CAD build for the part. Positions are in the model's coordinates, mm. Give positions to 0.01 mm unless a question says otherwise; leave off trailing zeros. Write each loop counter-clockwise with the first axis right and the second up, starting at its lowest first coordinate (ties: lowest second). Pieces come first, ordered by that corner, then holes. Notation, with made-up numbers: (54.5, 21.5) -> (71.5, 21.5) arc R31 ccw to (71.5, 49.5) -> close; hole circle Ø3 at (82.25, -31). An arc over 180 degrees is marked (long way). Answer as a JSON object with one key per item and string values.
Autodesk Inventor part; units mm, degrees
ref_plane "YZ Plane" through (0, 0, 0) normal (1, 0, 0) x (0, 1, 0)
ref_plane "XZ Plane" through (0, 0, 0) normal (0, 1, 0) x (-1, 0, 0)
ref_plane "XY Plane" through (0, 0, 0) normal (0, 0, 1) x (1, 0, 0)
sketch "Sketch1" plane through (0, 0, 0) normal (0, 1, 0) x (-1, 0, 0)
  line L0 (0, 0) -> (254, 0)
  line L1 (0, -25.4) -> (254, -25.4)
  line L2 (0, 25.4) -> (254, 25.4)
  circle A0 centre (254, 0) radius 25.4
  circle A1 centre (0, 0) radius 25.4
  circle A2 centre (254, 0) radius 14.2875
  circle A3 centre (0, 0) radius 14.2875
  line L3 (76.2, 0) -> (-84.1335, 0)
  line L4 (121.5695, -25.4) -> (-84.1335, -25.4)
  line L5 (40.7781, 25.4) -> (-84.1335, 25.4)
  circle A4 centre (-84.1335, 0) radius 25.4
  line L6 (152.4, 0) -> (371.644, 165.4814)
  line L7 (143.8902, 25.4) -> (356.342, 185.7548)
  line L8 (228.214, 25.4) -> (386.946, 145.208)
  circle A5 centre (371.644, 165.4814) radius 25.4
  circle A6 centre (371.644, 165.4814) radius 14.2875
  circle A7 centre (-34.5114, 79.1283) radius 25.4
  line L9 (53.0811, 0) -> (-34.5114, 79.1283)
  line L10 (13.4025, 70.0738) -> (8.7814, 74.2485)
  line L11 (-4.2871, 17.5951) -> (-21.5461, 33.1863)
  line L12 (-9.1867, 81.0827) -> (-4.2871, 17.5951)
  line L13 (-17.4847, 97.9764) -> (13.4025, 70.0738)
  line L14 (-34.5114, 79.1283) -> (371.644, 165.4814)
  line L15 (366.3617, 190.3261) -> (-88.4526, 93.6275)
  line L16 (-88.4526, 93.6275) -> (19.2621, -3.6785)
  line L17 (409.5559, 199.5096) -> (-88.4526, 93.6275)
  line L18 (-88.4526, 93.6275) -> (-12.9269, 25.4)
  line L19 (419.8284, 149.7582) -> (19.4297, 64.629)
  line L20 (19.4297, 64.629) -> (62.855, 25.4)
  circle A8 centre (-34.5114, 79.1283) radius 12.7
  line L21 (19.4297, 64.629) -> (-88.4526, 93.6275)
  circle A9 centre (-59.0407, 85.7217) radius 3.4925
  circle A10 centre (-9.9821, 72.5349) radius 3.4925
  line L22 (99.5982, 0) -> (99.5982, -97.1111)
  line L23 (99.5982, -97.1111) -> (33.9277, 0)
  line L24 (99.5982, -97.1111) -> (168.3997, 0)
  line L25 (197.5982, 128.4774) -> (41.1424, 225.5805)
  line L26 (41.1424, 225.5805) -> (83.0141, 104.1155)
  line L27 (41.1424, 225.5805) -> (300.5341, 150.3627)
  point P0 (107.1023, -119.4279)
  point P1 (121.5695, -25.4)
  point P2 (2.9551, -25.4)
  point P3 (143.8902, 25.4)
  point P4 (258.2652, 25.0393)
  point P5 (0, 25.4)
  point P6 (16.3526, 37.9742)
  point P7 (0.338, 25.4)
  point P8 (70.7471, 25.4)
  point P9 (4.9006, 69.9742)
  point P10 (-10.4414, 23.1547)
  point P11 (17.5299, 80.8522)
  point P12 (265.0526, 116.8512)
  point P13 (396.2371, 108.5044)
  point P14 (-39.7937, 103.973)
  point P15 (-57.9044, 89.0242)
  point P16 (-51.5382, 60.2802)
  point P17 (-59.7133, 82.2946)
  point P18 (20.6525, 89.1934)
  point P19 (16.5095, 73.5132)
  point P20 (-9.3095, 75.962)
  point P21 (-15.6634, 62.1015)
  point P22 (160.2581, 29.4846)
  point P23 (-11.1184, 69.2324)
  point P24 (382.4437, 141.8098)
  point P25 (376.9262, 140.6367)
  point P26 (323.7481, 129.3305)
  point P27 (186.0521, 25.4)
  point P28 (24.9641, 25.4)
  point P29 (-4.2871, 17.5951)
  point P30 (-12.9269, 25.4)
  point P31 (4.4913, 25.4)
  point P32 (231.3112, 11.4183)
  point P33 (277.9303, 8.5148)
  point P34 (351.3706, 150.1794)
  point P35 (312.9484, 153.0021)
  point P36 (346.7993, 160.1992)
  point P37 (-88.4526, 93.6275)
  point P38 (-2.1293, 19.9838)
  point P39 (-7.1267, 54.3898)
  point P40 (-9.6667, 84.4105)
  point P41 (371.644, 165.4814)
  point P42 (278.63, 6.2067)
  point P43 (230.4586, 9.5373)
  point P44 (-4.8895, 25.4)
  point P45 (60.8476, 25.4)
  point P46 (229.1391, 5.2053)
  point P47 (-12.9269, 25.4)
  point P48 (1.0288, 25.4)
  point P49 (-4.8534, 24.932)
  point P50 (-87.4545, 179.42)
  point P51 (74.6737, 128.31)
  point P52 (248.8661, 165.3452)
  dimension "d0" = 25.4
  dimension "d1" = 25.4
  dimension "d2" = 28.575
  dimension "d3" = 28.575
  dimension "d6" = 254
  dimension "d7" = 76.2
  dimension "d8" = 25.4
  dimension "d9" = 25.4
  dimension "d11" = 50.8
  dimension "d13" = 25.4
  dimension "d14" = 25.4
  dimension "d15" = 50.8
  dimension "d16" = 101.6
  dimension "d18" = 28.575
  dimension "d23" = 50.8
  dimension "d24" = 25.4
  dimension "d25" = 25.4
  dimension "d26" = 25.4
  dimension "d27" = 25.4
  dimension "d28" = 25.4
  dimension "d29" = 25.4
  dimension "d30" = 6.985
  dimension "d31" = 6.985
extrude "Extrusion1" add sketch "Sketch1" along normal blind 6.35 contours L3 A3 L16 L0 | L0 A3 L3 | A3 L16 L0 | L0 A1 L3 A3 | L3 A1 L11 L16 A3 | L16 A3 L12 A1 L0 | L16 A3 | L3 A4 L5 L11 A1 | A1 L4 A4 L3 | A1 L2 L9 L0 | L0 L23 L1 A1 | L11 A1 L12 | L11 L5 L12 A1 | A4 | L0 L22 L1 L23 | L5 L12 L9 L2 | A1 L12 L5 | L11 L16 A7 L9 L12 L5 | L9 L2 L6 L0 | L9 L12 A10 L21 L20 L2 | L22 L0 L24 L1 | L9 A7 A10 L12 | L16 L21 A9 A7 | A7 A9 L21 A8 L9 | L24 L0 A0 L1 | L20 L19 L7 L2 | L9 A8 L21 A10 A7 | A10 A7 L21 L12 | L12 L21 A10 | A9 L21 A7 | A7 L21 A9 | L15 A7 A9 L21 | L6 L2 A0 L0 | A2 | A0 | L7 L19 L6 L2 | L21 A10 L12 A7 L14 L7 L19 | A10 L21 A7 | A8 L21 L9 | L9 L21 A8 | L21 A7 A10 L12 | L12 A10 L21 | L21 A9 A7 | A7 A9 L21 | A9 A7 L14 A8 L21 | L15 L26 L14 L13 A7 | L6 L19 L8 L2 | L7 L14 A5 L6 L19 | L21 A10 A7 | L21 A8 L14 A7 A10 | L21 A8 L14 | L14 A8 L21 | A10 A7 L12 | L13 L14 A7 | L26 L25 L15 | L15 L25 L14 L26 | L6 A5 L19 | L14 L27 L15 A5 L7 | L7 A5 L14 | L25 L27 L15 | L15 L27 L14 L25 | L19 A5 L8 | A5 L14 A6 L6 | L6 A6 L14 A5 | A6 L14 L6 | L6 L14 A6
extrude "Extrusion2" cut sketch "Sketch1" along normal through all contours L3 A3 L16 L0 | L0 A3 L3 | L16 A3 | L20 L19 L7 L2 | A10 A7 L21 L12 | L12 L21 A10 | A7 L21 A9 | A2 | A10 L21 A7 | A8 L21 L9 | L9 L21 A8 | L21 A7 A10 L12 | L12 A10 L21 | A7 A9 L21 | L21 A10 A7 | L21 A8 L14 | L14 A8 L21 | A6 L14 L6 | L6 L14 A6 picked at (-58.0988, 84.8098) picked at (-57.7672, 86.0943)
fillet "Fillet2" radius 19.05 1 edges at (88.4526, 3.175, 93.6275)
equation "\"d0\" = d1"
properties part number "intake-1"
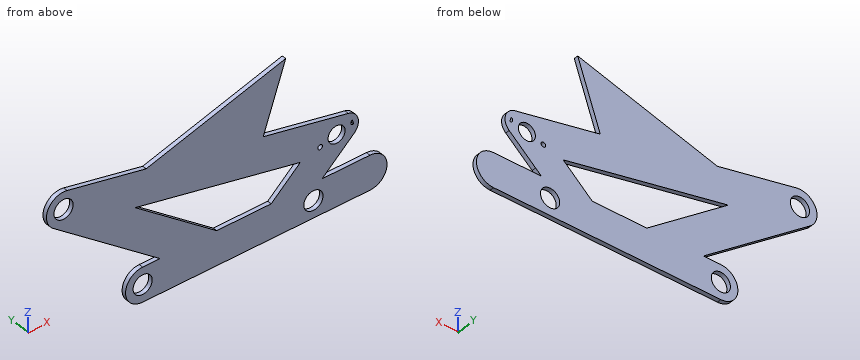
1) Slice it at A-A (z = 0). List the corners of the cut face in (x, y), then the cut area to 3 significant figures.
Model answer:
{"outline": "(-279.4, 0) -> (-268.29, 0) -> (-268.29, 6.35) -> (-279.4, 6.35) -> close; (-239.71, 0) -> (-14.29, 0) -> (-14.29, 6.35) -> (-239.71, 6.35) -> close; (14.29, 0) -> (109.53, 0) -> (109.53, 6.35) -> (14.29, 6.35) -> close", "area": "2,110 mm2"}
2) Slice it at B-B (x = -105.5). List the corners of the cut face in (y, z), then the cut area to 3 significant figures.
Model answer:
{"outline": "(0, -25.4) -> (6.35, -25.4) -> (6.35, 25.4) -> (0, 25.4) -> close; (0, 82.93) -> (6.35, 82.93) -> (6.35, 206.92) -> (0, 206.92) -> close", "area": "1,110 mm2"}
3) Slice it at D-D (x = 28). List the corners of the cut face in (y, z), then the cut area to 3 significant figures.
Model answer:
{"outline": "(0, -25.4) -> (6.35, -25.4) -> (6.35, 25.4) -> (0, 25.4) -> close; (0, 39.02) -> (6.35, 39.02) -> (6.35, 68.22) -> (0, 68.22) -> close; (0, 90.03) -> (6.35, 90.03) -> (6.35, 106.48) -> (0, 106.48) -> close", "area": "612 mm2"}
4) Slice it at C-C (y = 5.25). State how many separate pieces and enclosed holes the cut face has, then the cut area to 3 significant figures.
Model answer:
{"separate pieces": "1", "enclosed holes": "7", "area": "60,400 mm2"}
5) Pin check, flat tips, straight feed: pin 1 (1.5 mm diameter, centred on x = -278, z = 101.5, fed in from -Y); pin 2 (1.9 mm diameter, centred on x = -241, y = 4.5, fed in from +Z); pin 3 (1.5 mm diameter, centred on y = 4.5, z = 44.5, fed in from -X); pin 4 (2 mm diameter, centred on y = 3.5, z = 59.5, fed in from -X). Stop position of each tip, or through.
Model answer:
{"pin 1": "stops at y = 0", "pin 2": "stops at z = 167.9", "pin 3": "stops at x = -254.51", "pin 4": "stops at x = -274.72"}
6) Wall check: probe 1 along X at (y, z) = (3.25, 0); probe 2 along Z at (x, y) = (-251.5, 1); probe 3 along Z at (x, y) = (12, 4.75). Give the ranges that are in metal, low to high.
Model answer:
{"probe 1": "x = -279.4 to -268.29, -239.71 to -14.29, 14.29 to 109.53", "probe 2": "z = -25.4 to -14.07, 14.07 to 25.4, 42.98 to 106.62, 113.97 to 165.91", "probe 3": "z = -25.4 to -7.75, 7.75 to 69.68, 75.39 to 109.88"}
